Source: CAD feature listing. Evaluate the final solid. Frame: model axes, mm. Round coordinates to 2 decimals unless told otherwise and drop trailing zeros. Order: outer loops, then holes, each group sorted by start corner. A loop starts at its lowest first (then second) coordinate and runs counter-clockwise, first axis right, second up. Notation, with made-up numbers: (16.5, 58) - (57.5, 58) arc R7 ccw to (57.5, 65) - close; hole circle Ø8 at (25, 80.25). An arc over 180 degrees is marked (long way). Return JSON: item names as keys, results as strings. Group by question number.
1) Section C-C, the plane y = 5. Return loops of the section in (x, z), plus the area to 3 significant figures.
2) Ray query, line 1 (Y direction, x = 2.4, z = -5); line 2 (Z direction, x = 1.8, y = 5.25); line 3 (Y direction, x = 1.2, z = -8.5). Return the intervals inside material, ascending. Write a range as from..to.
3) Section B-B, the plane z = -27. Return loops of the section in (x, y), plus the area to 3 significant figures.
4) Section A-A, the plane x = 1.65. Return loops of the section in (y, z), plus the area to 3 significant figures.
5) Contact query for flat-ended pins moving along their axis: P1, Ø0.9, axis at x = 1.5, z = -16.5, coming from the +Y side; P2, Ø1.5, axis at x = 0.5, z = -40.5, coming from the +Y side; P3, Ø1.5, axis at x = 1, z = -42, coming from the +Y side. Output: stop coordinate, or through.
6) Section D-D, the plane z = -17. Return loops of the section in (x, y), plus the area to 3 significant figures.
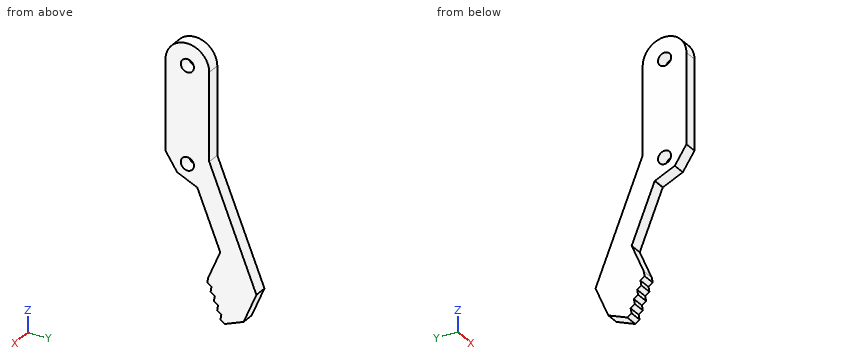
```python
from build123d import *

# Parameters (mm, degrees)
SKETCH1_R           = 5
SKETCH1_R_2         = 1.5
BOSS_EXTRUDE1_DEPTH = 3
BOSS_EXTRUDE2_DEPTH = 3
CUT_EXTRUDE2_DEPTH  = 4
CUT_EXTRUDE3_DEPTH  = 10


with BuildPart() as part:
    # Sketch1 → Boss-Extrude1 (new body)
    with BuildSketch(Plane(origin=(0, 0, 0), x_dir=(0, 0, -1), z_dir=(1, 0, 0))):
        with Locations((5, 5)):
            Circle(SKETCH1_R)
        with Locations((5, 5)):
            Circle(SKETCH1_R_2, mode=Mode.SUBTRACT)
        with BuildLine():
            ThreePointArc((10, 5), (8.535533906, 1.464466094), (5, 0))
            Line((5, 0), (27, 0))
            ThreePointArc((27, 0), (22, 5), (27, 10))
            Line((27, 10), (5, 10))
            ThreePointArc((5, 10), (8.535533906, 8.535533906), (10, 5))
        make_face()
        with Locations((27, 5)):
            Circle(SKETCH1_R)
        with Locations((27, 5)):
            Circle(SKETCH1_R_2, mode=Mode.SUBTRACT)
    extrude(amount=BOSS_EXTRUDE1_DEPTH)

    # Sketch2 → Boss-Extrude2 (add)
    with BuildSketch(Plane(origin=(3, 0, 0), x_dir=(0, 0, -1), z_dir=(1, 0, 0))):
        with BuildLine():
            ThreePointArc((27, 10), (29.694507461, 9.21184396), (31.53953799, 7.095851816))
            Line((31.53953799, 7.095851816), (31.610157793, 7.262674791))
            Line((31.610157793, 7.262674791), (44.585599673, 12.519851602))
            Line((44.585599673, 12.519851602), (51.097249205, 9.763328363))
            Line((51.097249205, 9.763328363), (60.365421977, 13.518454657))
            Line((60.365421977, 13.518454657), (56.610295683, 22.786627428))
            Line((56.610295683, 22.786627428), (25.051124858, 10))
            Line((25.051124858, 10), (27, 10))
        make_face()
        Polygon((60.365421977, 13.518454657), (51.097249205, 9.763328363), (51.333822162, 9.179433479), (60.601994933, 12.934559772), align=None)
    extrude(amount=-BOSS_EXTRUDE2_DEPTH)

    # Sketch4 → Cut-Extrude2 (cut, through all)
    with BuildSketch(Plane(origin=(3, 0, 0), x_dir=(0, 0, -1), z_dir=(1, 0, 0))):
        Polygon((56.610295683, 22.786627428), (51.684261855, 20.790777803), (58.606145308, 17.8605936), align=None)
    extrude(amount=-CUT_EXTRUDE2_DEPTH, mode=Mode.SUBTRACT)

    # Sketch5 → Cut-Extrude3 (cut)
    with BuildSketch(Plane(origin=(3, 0, 0), x_dir=(0, 0, -1), z_dir=(1, 0, 0))):
        with BuildLine():
            ThreePointArc((27, 0), (31.21184396, 2.305492539), (31.53953799, 7.095851816))
            Line((31.53953799, 7.095851816), (29.583779735, 2.664986829))
            Line((29.583779735, 2.664986829), (25.539598719, 0))
            Line((25.539598719, 0), (27, 0))
        make_face()
        Polygon((52.260639439, 9.554946108), (51.097249205, 9.763328363), (51.333822162, 9.179433479), align=None)
        Polygon((52.95088376, 10.514353622), (52.260639439, 9.554946108), (54.114273993, 10.305971367), align=None)
        Polygon((54.804518314, 11.265378881), (54.114273993, 10.305971367), (55.967908548, 11.056996626), align=None)
        Polygon((56.658152868, 12.01640414), (55.967908548, 11.056996626), (57.821543102, 11.808021884), align=None)
        Polygon((58.511787422, 12.767429398), (57.821543102, 11.808021884), (59.675177656, 12.559047143), align=None)
        Polygon((60.365421977, 13.518454657), (59.675177656, 12.559047143), (60.601994933, 12.934559772), align=None)
    extrude(amount=-CUT_EXTRUDE3_DEPTH, mode=Mode.SUBTRACT)


solid = part.part
```
Geometry check:
{
 "1": {"outline": "(0, -30.61) - (3, -30.61) - (3, -28.5) - (0, -28.5) - close; (0, -25.5) - (3, -25.5) - (3, -6.5) - (0, -6.5) - close; (0, -3.5) - (3, -3.5) - (3, 0) - (0, 0) - close", "area": "73.8 mm2"},
 "2": {"line 1": "0..3.5, 6.5..10", "line 2": "-30.72..-28.48, -25.52..-6.48, -3.52..-0.01", "line 3": "0..10"},
 "3": {"outline": "(0, 0.96) - (3, 0.96) - (3, 3.5) - (0, 3.5) - close; (0, 6.5) - (3, 6.5) - (3, 10.79) - (0, 10.79) - close", "area": "20.5 mm2"},
 "4": {"outline": "(0, -25.54) - (2.66, -29.58) - (7.1, -31.54) - (7.26, -31.61) - (12.52, -44.59) - (9.76, -51.1) - (9.55, -52.26) - (10.51, -52.95) - (10.31, -54.11) - (11.27, -54.8) - (11.06, -55.97) - (12.02, -56.66) - (11.81, -57.82) - (12.77, -58.51) - (12.56, -59.68) - (13.52, -60.37) - (17.86, -58.61) - (20.79, -51.68) - (10, -25.05) - (10, -5) arc R5 ccw to (0, -5) - close; hole circle Ø3 at (5, -27); hole circle Ø3 at (5, -5)", "area": "476 mm2"},
 "5": {"P1": "y = 10", "P2": "y = 16.56", "P3": "y = 17.17"},
 "6": {"outline": "(0, 0) - (3, 0) - (3, 10) - (0, 10) - close", "area": "30.0 mm2"}
}
